from build123d import *

# Parameters (mm, degrees)
F1_DEPTH      = 1.5
F1_DEPTH_BACK = 1.5
F3_DEPTH      = 4
F3_DEPTH_BACK = 4
F5_DEPTH      = 3
F5_DEPTH_BACK = 3
F6_R          = 2.5
F6_R_2        = 2.75
F7_DEPTH      = 4.001
F7_DEPTH_BACK = 4.001
F8_T4_DEPTH   = 22.9123439264
F8_T10_DEPTH  = 21.8550350011
F8_T16_DEPTH  = 21.8550350011
F8_T22_DEPTH  = 22.9123439264
F10_R         = 1
F11_DEPTH     = 6.3649610307


# Not quite as in the source:
# - a fillet or chamfer that OpenCascade refuses, or shapes differently, is made with other operations: its cross-section is extruded or revolved along the edge and cut away or added


with BuildPart() as f1:
    # F0 (on Front) → F1 (new body, two sides)
    with BuildSketch(Plane.XZ) as f1_sk:
        with BuildLine():
            Line((16.4318181818, 4.4994834414), (-16.5606060606, 3.9995408368))
            ThreePointArc((-16.5606060606, 3.9995408368), (-20.5, 0), (-16.5606060606, -3.9995408368))
            Line((-16.5606060606, -3.9995408368), (16.4318181818, -4.4994834414))
            ThreePointArc((16.4318181818, -4.4994834414), (21, 0), (16.4318181818, 4.4994834414))
        make_face()
    extrude(amount=F1_DEPTH)
    extrude(f1_sk.sketch, amount=-F1_DEPTH_BACK)

    # F2 (on Front) → F3 (join, two sides)
    with BuildSketch(Plane.XZ) as f3_sk:
        with BuildLine():
            Line((-12.5, 4.0610722343), (-16.5606060606, 3.9995408368))
            ThreePointArc((-16.5606060606, 3.9995408368), (-20.5, 0), (-16.5606060606, -3.9995408368))
            Line((-16.5606060606, -3.9995408368), (-12.5, -4.0610722343))
            Line((-12.5, -4.0610722343), (-12.5, 4.0610722343))
        make_face()
    extrude(amount=F3_DEPTH)
    extrude(f3_sk.sketch, amount=-F3_DEPTH_BACK)

    # F4 (on Front) → F5 (join, two sides)
    with BuildSketch(Plane.XZ) as f5_sk:
        with BuildLine():
            Line((16.4318181818, 4.4994834414), (12, 4.4323269722))
            Line((12, 4.4323269722), (12, -4.4323269722))
            Line((12, -4.4323269722), (16.4318181818, -4.4994834414))
            ThreePointArc((16.4318181818, -4.4994834414), (21, 0), (16.4318181818, 4.4994834414))
        make_face()
    extrude(amount=F5_DEPTH)
    extrude(f5_sk.sketch, amount=-F5_DEPTH_BACK)

    # F6 (on Front) → F7 (cut, two sides)
    with BuildSketch(Plane.XZ) as f7_sk:
        with Locations((-16.5, 0)):
            Circle(F6_R)
        with Locations((16.5, 0)):
            Circle(F6_R_2)
    extrude(amount=-F7_DEPTH, mode=Mode.SUBTRACT)
    extrude(f7_sk.sketch, amount=F7_DEPTH_BACK, mode=Mode.SUBTRACT)

    # F8: fillet of radius 3 on 4 edges, made by hand


with BuildPart() as f8_tool2:
    # F8_s3 → F8_t4 (new body)
    with BuildSketch(Plane.XY.offset(11.4561719632)):
        with BuildLine():
            ThreePointArc((-12.5, -4), (-11.4784517816, -2.2087121525), (-9.5419601084, -1.5))
            Line((-9.5419601084, -1.5), (-12.5, -1.5))
            Line((-12.5, -1.5), (-12.5, -4))
        make_face()
    extrude(amount=-F8_T4_DEPTH)

    split(bisect_by=Plane(origin=(-0.0643939394, 0, -4.2495121391), x_dir=(0, 1, 0), z_dir=(0.0151515152, 0, 0.9998852092)), keep=Keep.TOP)

    split(bisect_by=Plane(origin=(-0.0643939394, 0, 4.2495121391), x_dir=(0, 1, 0), z_dir=(0.0151515152, 0, -0.9998852092)), keep=Keep.TOP)


with BuildPart() as f1_1:
    add(f1.part)

    # F8_t1: union F8_tool2
    add(f8_tool2.part)


with BuildPart() as f8_tool8:
    # F8_s9 → F8_t10 (new body)
    with BuildSketch(Plane.XY.offset(-10.9275175005)):
        with BuildLine():
            ThreePointArc((9.4019237886, -1.5), (10.9019237886, -1.9019237886), (12, -3))
            Line((12, -3), (12, -1.5))
            Line((12, -1.5), (9.4019237886, -1.5))
        make_face()
    extrude(amount=F8_T10_DEPTH)

    split(bisect_by=Plane(origin=(-0.0643939394, 0, -4.2495121391), x_dir=(0, 1, 0), z_dir=(0.0151515152, 0, 0.9998852092)), keep=Keep.TOP)

    split(bisect_by=Plane(origin=(-0.0643939394, 0, 4.2495121391), x_dir=(0, 1, 0), z_dir=(0.0151515152, 0, -0.9998852092)), keep=Keep.TOP)


with BuildPart() as f1_2:
    add(f1_1.part)

    # F8_t7: union F8_tool8
    add(f8_tool8.part)


with BuildPart() as f8_tool14:
    # F8_s15 → F8_t16 (new body)
    with BuildSketch(Plane.XY.offset(-10.9275175005)):
        with BuildLine():
            ThreePointArc((12, 3), (10.9019237886, 1.9019237886), (9.4019237886, 1.5))
            Line((9.4019237886, 1.5), (12, 1.5))
            Line((12, 1.5), (12, 3))
        make_face()
    extrude(amount=F8_T16_DEPTH)

    split(bisect_by=Plane(origin=(-0.0643939394, 0, -4.2495121391), x_dir=(0, 1, 0), z_dir=(0.0151515152, 0, 0.9998852092)), keep=Keep.TOP)

    split(bisect_by=Plane(origin=(-0.0643939394, 0, 4.2495121391), x_dir=(0, 1, 0), z_dir=(0.0151515152, 0, -0.9998852092)), keep=Keep.TOP)


with BuildPart() as f1_3:
    add(f1_2.part)

    # F8_t13: union F8_tool14
    add(f8_tool14.part)


with BuildPart() as f8_tool20:
    # F8_s21 → F8_t22 (new body)
    with BuildSketch(Plane.XY.offset(11.4561719632)):
        with BuildLine():
            ThreePointArc((-9.5419601084, 1.5), (-11.4784517816, 2.2087121525), (-12.5, 4))
            Line((-12.5, 4), (-12.5, 1.5))
            Line((-12.5, 1.5), (-9.5419601084, 1.5))
        make_face()
    extrude(amount=-F8_T22_DEPTH)

    split(bisect_by=Plane(origin=(-0.0643939394, 0, -4.2495121391), x_dir=(0, 1, 0), z_dir=(0.0151515152, 0, 0.9998852092)), keep=Keep.TOP)

    split(bisect_by=Plane(origin=(-0.0643939394, 0, 4.2495121391), x_dir=(0, 1, 0), z_dir=(0.0151515152, 0, -0.9998852092)), keep=Keep.TOP)


with BuildPart() as f1_4:
    add(f1_3.part)

    # F8_t19: union F8_tool20
    add(f8_tool20.part)

    # F10 (on face) → F11 (cut, through all)
    with BuildSketch(Plane(origin=(8.25, 0, 8.25), x_dir=(0.7071067812, 0, -0.7071067812), z_dir=(0.7071067812, 0, 0.7071067812))):
        with Locations((11.6672618896, 0)):
            Circle(F10_R)
    extrude(amount=F11_DEPTH, mode=Mode.SUBTRACT)


solid = f1_4.part
Can you work these out from the model? Positions are in its coordinate system, mm. A direction names the side the tool comes from. Give positions to 0.01 mm unless a question says otherwise; leave off trailing zeros. Order: outer loops, then holes, each group sorted by start corner. A loop starts at its lowest first (then second) coordinate and runs counter-clockwise, first axis right, second up. Notation, with made-up numbers: M -26,-30 L -2,-30 A30 cw -2,-2 Z; hole C 14.5,49 d5. An arc over 180 degrees is marked long. Use a Markdown table: item, result. Add a question column.
Item 1: Suppose I cut it at C-C (x = -11). List the corners of the cut face in (y, z) for me, then the cut area to 3 significant figures.
Item 2: Suppose I cut it at A-A (z = 0). List the corners of the cut face in (x, y) for me.
Item 3: Suppose I cut it at D-D (x = -4.5). List the corners of the cut face in (y, z) for me, then the cut area to 3 significant figures.
Item 4: We'd pull the mould along Z, two halves only. Please class faces 5 (the flat face through (0, 1.5, 0)), 6 (the cylindrical face through (18.282, 0.044, 3.195)), 7 (the cylindrical face through (-20.5, -0.1, 0.1)): +Z half, -Z half, draft (parallel to the pull), parting line (faces both ways), or undercut.
Item 5: For faces 1 (the flat face through (14, 3, -2)), 2 (the cylindrical face through (-11.456, 2.19, 0.057)), 3 (the cylindrical face through (10.9, -1.9, -0.1)), 4 (the flat face through (14, -3, -2)), which set-ups out of +Z, -Z, +X, -X, +Y, -Y let a thin tool reach every point of the face, with its end or its side?
Item 6: Will these pins go through, and if not, where does the flat tip stop? pin 1 (4.5 mm diameter, centred on x = 2, z = -1.5, fed in from -Y); pin 2 (4.5 mm diameter, centred on x = 15, z = 1, fed in from -Y); pin 3 (1.5 mm diameter, centred on x = 7, y = -0.5, fed in from +Z).
Item 7: Suppose I cut it at B-B (y = 2). List the corners of the cut face in (x, z) for me, then the cut area to 3 significant figures.
Item 8: If I drill on L1, parallel to Z at x = 16.5, y = -1.5; L2, parallel to Z at x = -16.5, y = 1.75; L3, parallel to X at y = -1.25, z = -0.75, over which ranges is the centre line in solid material (lowest first)? Write a range as [from, to].
Answer sheet:
| question | item | result |
|---|---|---|
| 1 | outline | M -1.88,-4.08 L 1.88,-4.08 L 1.88,4.08 L -1.88,4.08 Z |
| 1 | area | 30.7 mm² |
| 2 | outline | M -20.5,-4 L -19,-4 L -19,4 L -20.5,4 Z; M -14,-4 L -12.5,-4 A3 cw -9.54,-1.5 L 9.4,-1.5 A3 cw 12,-3 L 13.75,-3 L 13.75,3 L 12,3 A3 cw 9.4,1.5 L -9.54,1.5 A3 cw -12.5,4 L -14,4 Z; M 19.25,-3 L 21,-3 L 21,3 L 19.25,3 Z |
| 3 | outline | M -1.5,-4.18 L 1.5,-4.18 L 1.5,4.18 L -1.5,4.18 Z |
| 3 | area | 25.1 mm² |
| 4 | face 5 | draft |
| 4 | face 6 | undercut |
| 4 | face 7 | parting line |
| 5 | face 1 | +Z, -Z, +X, +Y |
| 5 | face 2 | +Z, -Z, +Y |
| 5 | face 3 | +Z, -Z, -Y |
| 5 | face 4 | +Z, -Z, +X, -Y |
| 6 | pin 1 | stops at y = -1.5 |
| 6 | pin 2 | stops at y = -3 |
| 6 | pin 3 | stops at z = 4.37 |
| 7 | outline | M -16.56,-4 L -11.2,-4.08 L -11.2,4.08 L -16.56,4 A4 ccw Z; M 11.06,-4.42 L 16.43,-4.5 A4.5 ccw long 16.43,4.5 L 11.06,4.42 Z; hole C -16.5,0 d5; hole C 16.5,0 d5.5 |
| 7 | area | 105 mm² |
| 8 | L1 | z = [-4.5, -2.75], [2.75, 4.5] |
| 8 | L2 | z = [-4, -2.5], [2.5, 4] |
| 8 | L3 | x = [-20.43, -18.88], [-14.12, 13.85], [19.15, 20.94] |
